Design review of the part built by this model. Coordinates are the model's own, in mm. A direction names the side the tool comes from. Coordinates: 2 decimals unless noted, no trailing zeros. Write each loop counter-clockwise with the first axis right and the second up, starting at its lowest first coordinate (ties: lowest second). Pieces come first, ordered by that corner, then holes. Notation, with made-up numbers: (47.25, -24.5) - (74.25, -24.5) arc R12 ccw to (74.25, -13.5) - close; hole circle Ø5 at (-27, 15.25). An arc over 180 degrees is marked (long way). Answer as CSV lines item,"result". Start each with the question number.
Q1. We need section D-D (z = 16.5). Write out the cut boundary in (x, y), plus the area to 3 significant figures.
Q2. Mouldability with a two-part tool opening along X and no side actions: class faces 3 (the face through (-13, -79, 10)), 4 (the face through (-10, -79, 10)), 5 (the face through (15, -79, 0)), 6 (the face through (43, -79, 6)) as pulls with the +X half, pulls with the -X half, needs draft (parallel to the pull), parting line crosses it, or undercut.
Q3. We need section C-C (y = -50.5). Write out the cut boundary in (x, z).
Q4. Clearance check with a flat-ended pin moving along its axis: pin 1 (6 mm diameter, centred on x = 27, y = -46.5, fed in from +Z). State where the tip first meets the part, or that it passes through.
Q5. Machinability: for faces 1 (the face through (40, -79, 8)), 2 (the face through (14, 0, 2)), which of the approach directions +Z, -Z, +X, -X, +Y, -Y give a long, thin tool a straight path to every point of the face, cutting with its end or side? Answer none if there is none.
Q6. For line 1 along X through (y, z) = (-143.5, 7.5); line 2 along X through (y, z) = (-65.5, 14.75); line 3 along Z through (x, y) = (26.5, -146.5), list the stretches that pass through material, from the lowest coordinate up. Write a range as [from, to].
Q7. We need section B-B (x = 33.5). Write out the cut boundary in (y, z), plus the area to 3 significant figures.
Q8. We need section A-A (z = 6.5). Write out the cut boundary in (x, y).
from build123d import *

# Parameters (mm, degrees)
PAD_DEPTH   = 160
FILLET_R    = 2
FILLET001_R = 2
FILLET002_R = 0.9
FILLET003_R = 1


with BuildPart() as part:
    # Sketch → Pad (new body)
    with BuildSketch(Plane.XZ):
        Polygon((-13, 20), (-13, 0), (43, 0), (43, 13), (40, 13), (40, 3), (-10, 3), (-10, 20), align=None)
    extrude(amount=PAD_DEPTH)

    # Fillet
    fillet_edges = [part.edges().sort_by_distance(p)[0] for p in [
        (-11.5, -160, 20),
        (41.5, -160, 13),
        (-11.5, 0, 20),
        (41.5, 0, 13),
    ]]
    fillet(fillet_edges, radius=FILLET_R)

    # Fillet001
    fillet001_edges = [part.edges().sort_by_distance(p)[0] for p in [
        (43, -80, 13),
        (-10, -80, 20),
    ]]
    fillet(fillet001_edges, radius=FILLET001_R)

    # Fillet002
    fillet002_edges = [part.edges().sort_by_distance(p)[0] for p in [
        (40, -80, 13),
        (-13, -80, 20),
    ]]
    fillet(fillet002_edges, radius=FILLET002_R)

    # Fillet003
    fillet003_edges = [part.edges().sort_by_distance(p)[0] for p in [
        (14.45, -160, 0),
    ]]
    fillet(fillet003_edges, radius=FILLET003_R)


solid = part.part
Results list:
1,outline,"(-13, -159.1) arc R0.9 ccw to (-12.1, -160) - (-12, -160) arc R2 ccw to (-10, -158) - (-10, -2) arc R2 ccw to (-12, 0) - (-12.1, 0) arc R0.9 ccw to (-13, -0.9) - close"
1,area,"478 mm2"
2,face 3,"pulls with the -X half"
2,face 4,"undercut"
2,face 5,"needs draft"
2,face 6,"pulls with the +X half"
3,outline,"(-13, 1) arc R1 ccw to (-12, 0) - (42, 0) arc R1 ccw to (43, 1) - (43, 11) arc R2 ccw to (41, 13) - (40.9, 13) arc R0.9 ccw to (40, 12.1) - (40, 3) - (-10, 3) - (-10, 18) arc R2 ccw to (-12, 20) - (-12.1, 20) arc R0.9 ccw to (-13, 19.1) - close"
4,pin 1,"stops at z = 3"
5,face 1,"+Z, +Y, -Y"
5,face 2,"+Z, -Z, +X, -X, +Y"
6,line 1,"x = [-13, -10], [40, 43]"
6,line 2,"x = [-13, -10]"
6,line 3,"z = [0, 3]"
7,outline,"(-160, 1) arc R1 ccw to (-159, 0) - (-1, 0) arc R1 ccw to (0, 1) - (0, 3) - (-160, 3) - close"
7,area,"480 mm2"
8,outline,"(-13, -159.1) arc R0.9 ccw to (-12.1, -160) - (-12, -160) arc R2 ccw to (-10, -158) - (-10, -2) arc R2 ccw to (-12, 0) - (-12.1, 0) arc R0.9 ccw to (-13, -0.9) - close; (40, -159.1) arc R0.9 ccw to (40.9, -160) - (41, -160) arc R2 ccw to (43, -158) - (43, -2) arc R2 ccw to (41, 0) - (40.9, 0) arc R0.9 ccw to (40, -0.9) - close"
